Job drawing, mm, ordinate dimensions from the low corner. One solid piece. Give positions to 0.01 mm unless a question says otherwise; leave off trailing zeros. Loops run counter-clockwise (first coordinate to the right, second up) from the corner with the lowest first, then second, coordinate; pieces in that order, holes last. Notation, with made-up numbers: (-19.5, -36.5) - (21.5, -36.5) arc R32 cw to (21.5, -9.5) - close; hole circle Ø8 at (6.25, 29). An arc over 180 degrees is marked (long way). Answer as CSV lines item,"result". Start each with the question number.
Item 1: Pin check, flat tip, straight feed: pin 1 (0.5 mm diameter, centred on x = 14.5, z = 0.5, fed in from -Y). Stop position of the tip, or through.
Item 2: Pull direction X, two halves, no side cores. Call the marked faces 1, 2 and 3: pulls with the +X half, pulls with the -X half, needs draft (parallel to the pull), parting line crosses it, or undercut.
Item 3: Saw through at C-C on y = 5.5. Give the cut face in (x, z), plus the area to 3 significant figures.
Item 4: Saw through at D-D on y = 4.75. Give the cut face in (x, z).
Item 5: Saw through at A-A on x = 14.25. Give the cut face in (y, z).
Item 6: Drill centre lines: L1, parallel to X at y = 4, z = 0.25; L2, parallel to Y at x = 3.5, z = 0.4; L3, parallel to X at y = 1.5, z = 0.45. Where is each one in solid material? Low to high. Write a range as from..to.
Item 7: Saw through at B-B on z = 0.3. Give the cut face in (x, y), plus the area to 3 significant figures.
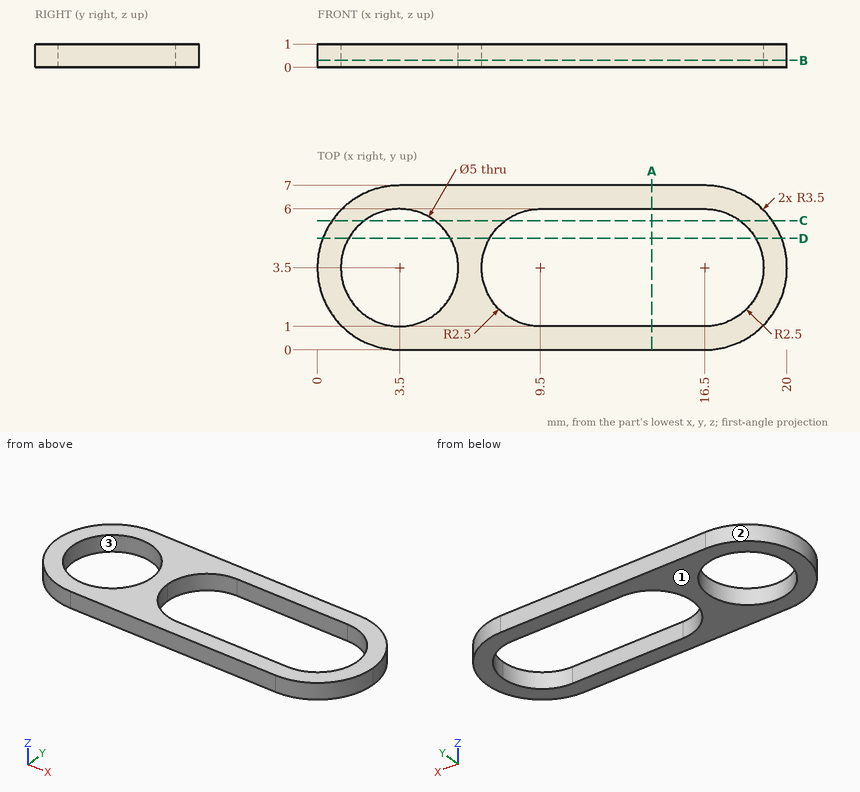
Responses:
1,pin 1,"y = 0"
2,face 1,"needs draft"
2,face 2,"pulls with the -X half"
2,face 3,"undercut"
3,outline,"(0.63, 0) - (2, 0) - (2, 1) - (0.63, 1) - close; (5, 0) - (8, 0) - (8, 1) - (5, 1) - close; (18, 0) - (19.37, 0) - (19.37, 1) - (18, 1) - close"
3,area,"5.74 mm2"
4,outline,"(0.23, 0) - (1.33, 0) - (1.33, 1) - (0.23, 1) - close; (5.67, 0) - (7.33, 0) - (7.33, 1) - (5.67, 1) - close; (18.67, 0) - (19.77, 0) - (19.77, 1) - (18.67, 1) - close"
5,outline,"(0, 0) - (1, 0) - (1, 1) - (0, 1) - close; (6, 0) - (7, 0) - (7, 1) - (6, 1) - close"
6,L1,"0.04..1.05, 5.95..7.05, 18.95..19.96"
6,L2,"0..1, 6..7"
6,L3,"0.63..2, 5..8, 18..19.37"
7,outline,"(3.5, 0) - (16.5, 0) arc R3.5 ccw to (16.5, 7) - (3.5, 7) arc R3.5 ccw to start; hole circle Ø5 at (3.5, 3.5); hole (9.5, 1) - (16.5, 1) arc R2.5 ccw to (16.5, 6) - (9.5, 6) arc R2.5 ccw to start"
7,area,"55.2 mm2"
